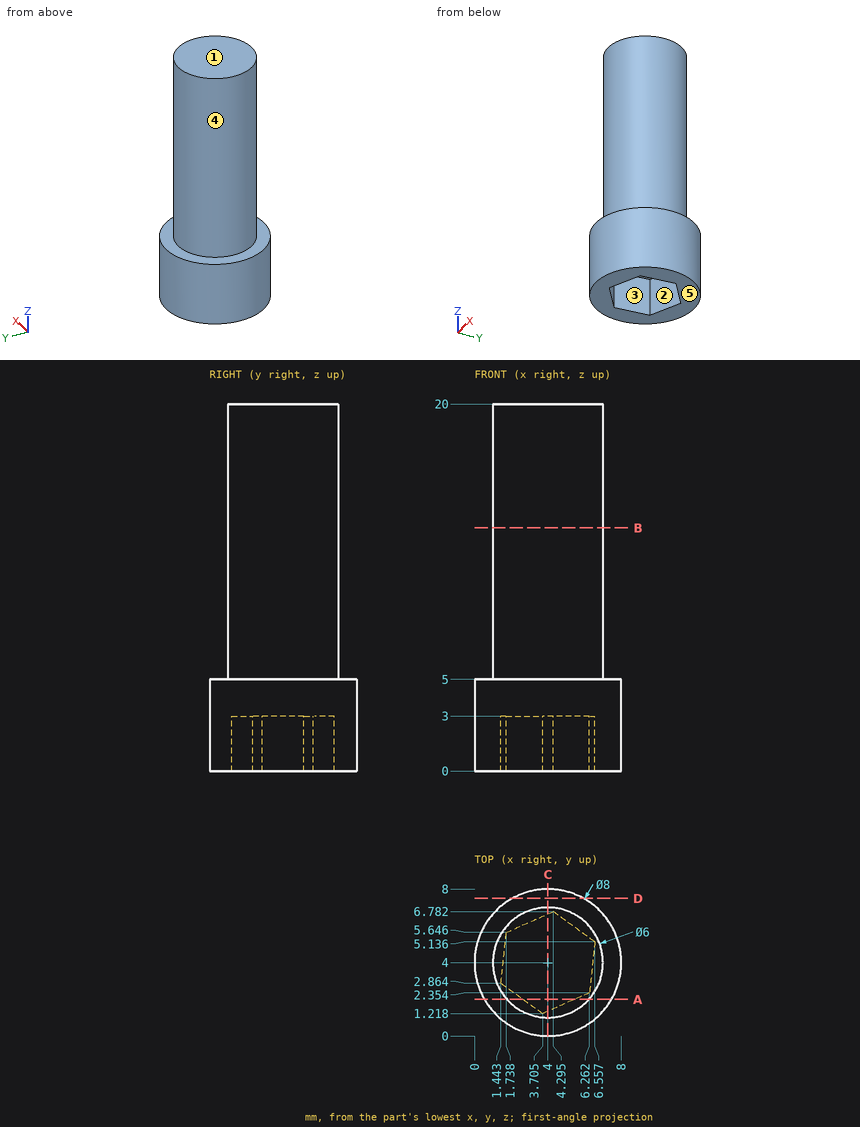
Input: dimensioned drawing with shaded views. Units: mm. Origin: part minimum x, y, z. A direction names the side the tool comes from. Round coordinates to 2 decimals unless told otherwise and drop trailing zeros. Order: outer loops, then holes, each group sorted by start corner. A loop starts at its lowest first (then second) coordinate and runs counter-clockwise, first axis right, second up.
1. Set-up query: the marked faces 1 and 2. Return all of +Z, -Z, +X, -X, +Y, -Y with unobstructed straight access to the full face (end or side cutting, diameter ignored); none if empty.
The answers:
face 1: +Z, +X, -X, +Y, -Y
face 2: -Z
2. Cut plane B-B, the plane z = 13.25. Output: boundary loops of the cut face in (x, y), then the cut area to 3 significant figures.
The answers:
outline: circle Ø6 at (4, 4)
area: 28.3 mm2
3. Cut plane C-C, the plane x = 4. Output: boundary loops of the cut face in (y, z), then the cut area to 3 significant figures.
The answers:
outline: (0, 0) - (1.35, 0) - (1.35, 3) - (6.65, 3) - (6.65, 0) - (8, 0) - (8, 5) - (7, 5) - (7, 20) - (1, 20) - (1, 5) - (0, 5) - close
area: 114 mm2
4. Cut plane A-A, the plane y = 2. Output: boundary loops of the cut face in (x, z).
The answers:
outline: (0.54, 0) - (2.63, 0) - (2.63, 3) - (5.47, 3) - (5.47, 0) - (7.46, 0) - (7.46, 5) - (6.24, 5) - (6.24, 20) - (1.76, 20) - (1.76, 5) - (0.54, 5) - close
5. Pin query (flat end, axial travel): P1, Ø1.5, axis at y = 7, z = 5, coming from the +X side; P2, Ø1.5, axis at x = 4.5, z = 15, coming from the +Y side; P3, Ø3, axis at x = 3, z = 10.5, coming from the -Y side. Return the tip coordinate at first contact, or that it passes through.
The answers:
P1: stops at x = 7.31
P2: stops at y = 7
P3: stops at y = 1
6. Cut plane D-D, the plane y = 7.5. Output: boundary loops of the cut face in (x, z).
The answers:
outline: (2.06, 0) - (5.94, 0) - (5.94, 5) - (2.06, 5) - close
7. Material intervals for line 1 (Z direction, x = 4.25, y = 4); line 2 (Z direction, x = 7, y = 6.25); line 3 (Y direction, x = 5.5, z = 1) (1 decimal), sorted ascending.
The answers:
line 1: z = 3 to 20
line 2: z = 0 to 5
line 3: y = 0.3 to 2, 5.9 to 7.7
8. Mould query, pull axis X, two halves, no side actions, for the marked faces 3, 4 and 5. Classes: released by +X, released by -X, zero draft, split by the parting line, or undercut.
The answers:
face 3: undercut
face 4: split by the parting line
face 5: zero draft
